Check sheet for the modelled part. Datum: model origin and axes. Units: mm. A direction names the side the tool comes from. Give positions to 0.01 mm unless a question says otherwise; leave off trailing zeros. Loops run counter-clockwise (first coordinate to the right, second up) from the corner with the lowest first, then second, coordinate; pieces in that order, holes last. Notation, with made-up numbers: M -36.5,69 L 21.5,69 A19 cw 21.5,78 Z; hole C 36,7.5 d8. An arc over 180 degrees is marked long. Put each result on its own line as item: value. Start each with the question number.
Autodesk Inventor part; units mm, degrees
ref_plane "YZ Plane" through (0, 0, 0) normal (1, 0, 0) x (0, 1, 0)
ref_plane "XZ Plane" through (0, 0, 0) normal (0, 1, 0) x (-1, 0, 0)
ref_plane "XY Plane" through (0, 0, 0) normal (0, 0, 1) x (1, 0, 0)
sketch "Sketch1" plane through (0, 0, 0) normal (0, 1, 0) x (-1, 0, 0)
  line L0 (25.15, 25.15) -> (-25.15, 25.15)
  line L1 (-25.15, 25.15) -> (-25.15, -25.15)
  line L2 (-25.15, -25.15) -> (25.15, -25.15)
  line L3 (25.15, -25.15) -> (25.15, 25.15)
  line L4 (25.15, 25.15) -> (-25.15, -25.15) construction
  line L5 (-25.15, 25.15) -> (25.15, -25.15) construction
  line L6 (30.15, 30.15) -> (-30.15, 30.15)
  line L7 (-30.15, 30.15) -> (-30.15, -30.15)
  line L8 (-30.15, -30.15) -> (30.15, -30.15)
  line L9 (30.15, -30.15) -> (30.15, 30.15)
  line L10 (30.15, 30.15) -> (-30.15, -30.15) construction
  line L11 (-30.15, 30.15) -> (30.15, -30.15) construction
  circle A0 centre (0, 0) radius 7.5
  circle A1 centre (0, 0) radius 9.65
  circle A2 centre (0, 0) radius 12.5
  line L12 (0, 0) -> (25.15, 0) construction
  line L13 (0, 0) -> (0, -25.15) construction
  dimension "d1" = 50.3
  dimension "d3" = 60.3
  dimension "d8" = 15
  dimension "d9" = 19.3
  dimension "d10" = 25
extrude "Extrusion1" add sketch "Sketch1" along normal blind 30 contours L9 L8 L7 L6
extrude "Extrusion2" add sketch "Sketch1" against normal blind 5 contours L3 L2 L1 L0 | L9 L8 L7 L6 | A1 | A2
extrude "Extrusion3" add sketch "Sketch1" along normal blind 6 contours A2
sketch "Sketch2" plane through (-30.15, 30, -30.15) normal (-1, 0, 0) x (0, 0, 1)
  line L0 (60.3, 0) -> (60.3, -35) construction
  line L1 (0, -35) -> (0, 0) construction
  circle A0 centre (45.15, -15) radius 2.25
  line L2 (30.15, -15) -> (45.15, -15) construction
  line L3 (30.15, -15) -> (15.15, -15) construction
  circle A1 centre (15.15, -15) radius 2.25
  line L4 (60.3, 0) -> (0, 0)
  line L5 (0, 0) -> (0, -30)
  line L6 (0, -30) -> (60.3, -30)
  line L7 (60.3, -30) -> (60.3, 0)
  line L8 (60.3, 0) -> (0, -30) construction
  line L9 (30.15, -15) -> (25.1861, -9.3551) construction
  point P0 (30.15, -30)
  dimension "d13" = 4.5
  dimension "d16" = 15
  dimension "d17" = 15
  dimension "d18" = 4.5
  dimension "d19" = 30
extrude "Extrusion4" cut sketch "Sketch2" against normal blind 65 contours A0 | A1
properties material "PBT Plastic"
Q1. Thickness scan on line 1 along Z through (x, y) = (-14, 27.5); line 2 along Y through (x, z) = (27.8, 15). Record the ranges inside material, lowest first. Write a range as [from, to].
Q2. Mould release check, pull along Z, two halves, no side actions. Record for faces 3 (the face through (27, 30, 0)), 4 (the face through (7.493, -2.465, 0.33)), 5 (the face through (0, 15, -25.15)), 6 (the face through (0, 12, 30.15)): pulls with the +Z half, pulls with the -Z half, needs draft (parallel to the pull), parting line crosses it, or undercut.
Q3. Section check B-B, the plane z = -15. Record the cut outline in (x, y), then the cut area to 4 significant figures.
Q4. Section check C-C, the plane x = 0. Record the cut outline in (y, z), then the cut area to 3 significant figures.
Q5. Section check A-A, the plane y = 3.5. Record the cut outline in (x, z), then the cut area to 3 significant figures.
Q6. Section check D-D, the plane z = 0. Record the cut outline in (x, y).
Q7. Depth check by flat-ended pin: P1, Ø4, axis at y = 15, z = 15, coming from the -X side; P2, Ø24, axis at x = 0, z = 0, coming from the +Y side; P3, Ø12, axis at x = 12.5, z = 18, coming from the +Y side; P4, Ø7, axis at y = 15, z = -15, coming from the -X side. Enter the tip coordinate at first touch or a pass-through.
Q8. Access from +Z, -Z, +X, -X, +Y, -Y to the whole of each face (thin tool, end or side, straight path). Record for faces 1 (the face through (-25.15, 15, 0)), 2 (the face through (-30.15, 12, 0)).
Found:
1. line 1: z = [-30.15, -25.15], [25.15, 30.15]
1. line 2: y = [-5, 12.75], [17.25, 30]
2. face 3: needs draft
2. face 4: undercut
2. face 5: undercut
2. face 6: pulls with the +Z half
3. outline: M -30.15,-5 L 30.15,-5 L 30.15,12.75 L 25.15,12.75 L 25.15,0 L -25.15,0 L -25.15,12.75 L -30.15,12.75 Z; M -30.15,17.25 L -25.15,17.25 L -25.15,30 L -30.15,30 Z; M 25.15,17.25 L 30.15,17.25 L 30.15,30 L 25.15,30 Z
3. area: 556.5 mm^2
4. outline: M -5,-30.15 L 30,-30.15 L 30,-25.15 L 0,-25.15 L 0,-12.5 L 6,-12.5 L 6,-9.65 L 0,-9.65 L 0,-7.5 L -5,-7.5 Z; M -5,7.5 L 0,7.5 L 0,9.65 L 6,9.65 L 6,12.5 L 0,12.5 L 0,25.15 L 30,25.15 L 30,30.15 L -5,30.15 Z
4. area: 561 mm^2
5. outline: M -30.15,-30.15 L 30.15,-30.15 L 30.15,30.15 L -30.15,30.15 Z; C 0,0 d25; hole M -25.15,-25.15 L 25.15,-25.15 L 25.15,25.15 L -25.15,25.15 Z; hole C 0,0 d19.3
5. area: 1,300 mm^2
6. outline: M -30.15,-5 L -7.5,-5 L -7.5,0 L -9.65,0 L -9.65,6 L -12.5,6 L -12.5,0 L -25.15,0 L -25.15,30 L -30.15,30 Z; M 7.5,-5 L 30.15,-5 L 30.15,30 L 25.15,30 L 25.15,0 L 12.5,0 L 12.5,6 L 9.65,6 L 9.65,0 L 7.5,0 Z
7. P1: passes through
7. P2: stops at y = 6
7. P3: stops at y = 0
7. P4: stops at x = -30.15
8. face 1: +Y
8. face 2: +Z, -Z, -X, +Y, -Y
